Job drawing, mm, ordinate dimensions from the low corner. One solid piece. A direction names the side the tool comes from. Round coordinates to 2 decimals unless told otherwise and drop trailing zeros. Loops run counter-clockwise (first coordinate to the right, second up) from the corner with the lowest first, then second, coordinate; pieces in that order, holes last.
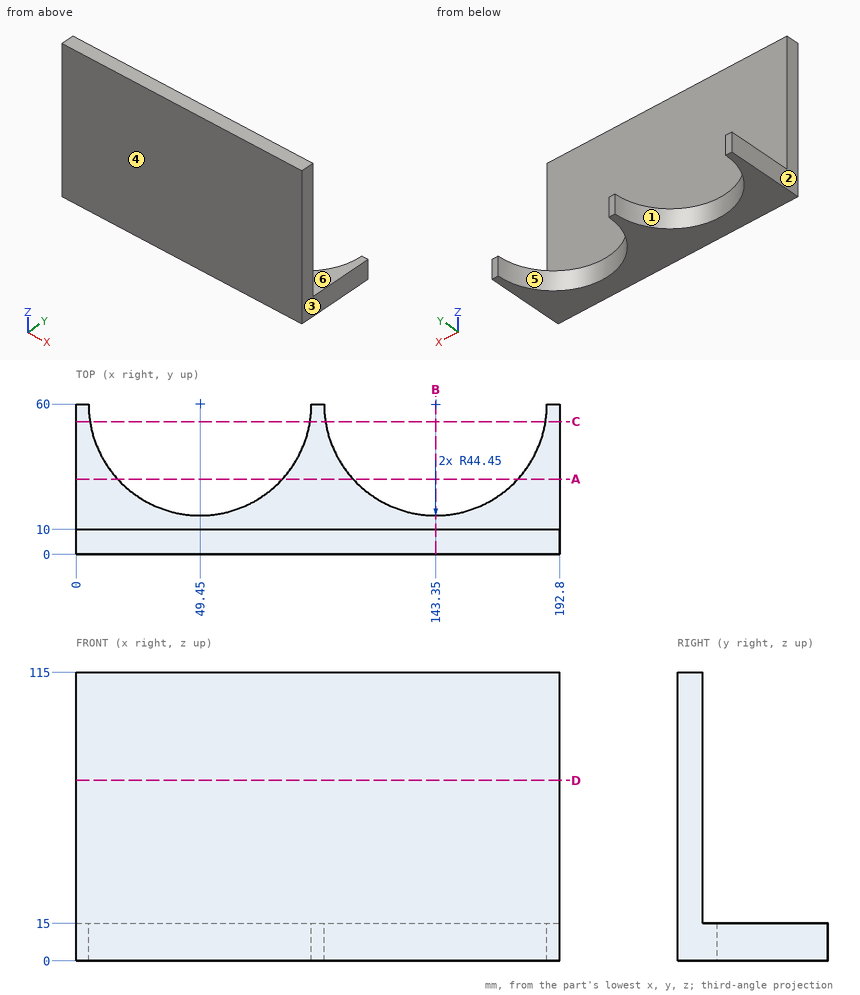
(1) Pull direction X, two halves, no side cores. Call the marked faces 1, 2, 3 and 4: +X half, -X half, draft (parallel to the pull), parting line (faces both ways), or undercut.
Responses:
face 1: undercut
face 2: -X half
face 3: +X half
face 4: draft
(2) Slice it at C-C on y = 53. List the corners of the cut face in (x, z).
Responses:
outline: (0, 0) - (5.55, 0) - (5.55, 15) - (0, 15) - close; (93.35, 0) - (99.45, 0) - (99.45, 15) - (93.35, 15) - close; (187.25, 0) - (192.8, 0) - (192.8, 15) - (187.25, 15) - close
(3) Probe line 1 (Y direction, x = 130.5, z = 97.5); line 2 (Z direction, x = 96, y = 27). List the from-to ranges inside material, lowest first.
Responses:
line 1: y = 0 to 10
line 2: z = 0 to 15
(4) Slice it at B-B on x = 143.35. List the corners of the cut face in (y, z).
Responses:
outline: (0, 0) - (15.55, 0) - (15.55, 15) - (10, 15) - (10, 115) - (0, 115) - close
(5) Slice it at D-D on z = 72. List the corners of the cut face in (x, y), plus the area to 3 significant figures.
Responses:
outline: (0, 0) - (192.8, 0) - (192.8, 10) - (0, 10) - close
area: 1,930 mm2
(6) Slice it at A-A on y = 30. List the corners of the cut face in (x, z).
Responses:
outline: (0, 0) - (16.65, 0) - (16.65, 15) - (0, 15) - close; (82.25, 0) - (110.55, 0) - (110.55, 15) - (82.25, 15) - close; (176.15, 0) - (192.8, 0) - (192.8, 15) - (176.15, 15) - close
(7) Pin check, flat tips, straight feed: P1, Ø4, axis at x = 35.5, z = 42.5, coming from the +Y side; P2, Ø1, axis at x = 61.5, z = 41.5, coming from the -Y side. Stop position of each tip, or through.
Responses:
P1: stops at y = 10
P2: stops at y = 0
(8) Which spindle directions (+Z, -Z, +X, -X, +Y, -Y) get a long thin tool onto all of the face, cutting with end or side? Do the marked faces 5 and 6. Say none if no direction does.
Responses:
face 5: +Z, -Z, +Y
face 6: +Z, +X, -X, +Y
